The model under review builds one solid part; all positions refer to its coordinate system, in mm. Face numbers are marked on the shaded views. A direction names the side the tool comes from. Round coordinates to 2 decimals unless told otherwise and drop trailing zeros. Loops run counter-clockwise (first coordinate to the right, second up) from the corner with the lowest first, then second, coordinate; pieces in that order, holes last. Notation, with made-up numbers: M 48.25,52.25 L 60.25,52.25 A15 cw 60.25,81.25 Z; hole C 85.5,13.25 d8. An arc over 180 degrees is marked long. Answer as a JSON object with one key per item and string values. Group by question number.
Item 1: To check wall thickness, follow line 1 (Y direction, x = 15.5, z = 11); line 2 (X direction, y = -7.5, z = -13.5); line 3 (Z direction, x = 50, y = -35). State the ranges of each line that lie inside material, in increasing order.
Item 2: Insertion check: P1, Ø20, axis at y = -24.43, z = 34.69, coming from the +X side; P2, Ø23, axis at x = 7.5, y = -34, coming from the +Z side; P3, Ø2, axis at x = 16, y = -1.5, coming from the +Z side. Each pin has a flat end and moves straight along its axis. Give the tip position at first contact, or say it passes through.
Item 3: Consider section A-A (z = -2.5). Give the boundary of the cut face in (x, y).
Item 4: The part is to be moulded in two halves that separate along X. For the marked faces 3, 4 and 5, say which applies: +X half, -X half, draft (parallel to the pull), parting line (faces both ways), or undercut.
Item 5: Consider section D-D (z = 33). Give the boundary of the cut face in (x, y).
Item 6: Tool access review of the marked faces 1 and 2: name each direction out of +Z, -Z, +X, -X, +Y, -Y from which nothing blocks a thin tool from reaching the whole face with its end or side.
Item 7: Consider section C-C (x = 9.5). Give the boundary of the cut face in (y, z), and give its area (3 significant figures).
Item 8: Consider section B-B (y = -28.5). Give the boundary of the cut face in (x, z).
```python
from build123d import *

# Parameters (mm, degrees)
F1_DEPTH = 50.8
F2_T     = -2.54
F3_R     = 6.296308
F4_DEPTH = 322.58


with BuildPart() as f1:
    # F0 (on Front) → F1 (new body)
    with BuildSketch(Plane.XZ):
        Polygon((-25.901856, 44.70605), (-47.471371, 44.70605), (-47.471371, -22.952178), (64.985082, -22.952178), (64.985082, 44.70605), (46.365242, 44.70605), (46.365242, 21.47734), (-25.901856, 21.47734), align=None)
    extrude(amount=F1_DEPTH)

    # F2
    f2_openings = [f1.faces().sort_by_distance(p)[0] for p in [
        (10.231693, -25.4, 21.47734),
        (-36.686613, -25.4, 44.70605),
        (55.675162, -25.4, 44.70605),
        (46.365242, -25.4, 33.091695),
        (-25.901856, -25.4, 33.091695),
    ]]
    offset(amount=F2_T, openings=f2_openings)

    # F3 (on face) → F4 (cut)
    with BuildSketch(Plane(origin=(-47.471371, 0, 0), x_dir=(0, -1, 0), z_dir=(-1, 0, 0))):
        with Locations((24.432799, 34.693193)):
            Circle(F3_R)
    extrude(amount=-F4_DEPTH, mode=Mode.SUBTRACT)


solid = f1.part
```
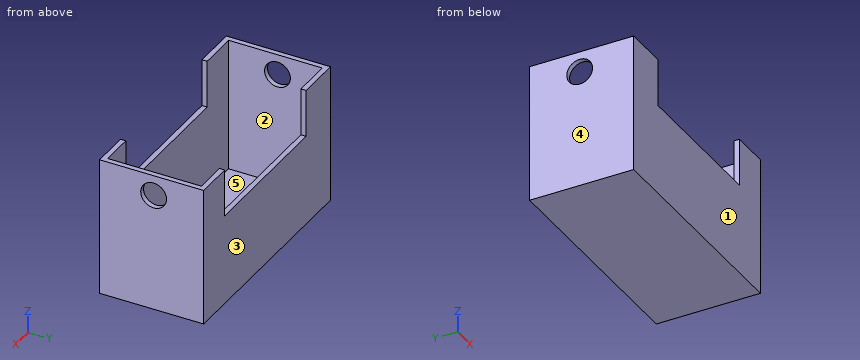
Geometry results:
{
 "1": {"line 1": "y = -50.8 to -48.26, -2.54 to 0", "line 2": "x = -47.47 to -44.93, 62.45 to 64.99", "line 3": "z = -22.95 to -20.41"},
 "2": {"P1": "stops at x = 64.99", "P2": "stops at z = -20.41", "P3": "stops at z = 21.48"},
 "3": {"outline": "M -47.47,-50.8 L 64.99,-50.8 L 64.99,0 L -47.47,0 Z; hole M -44.93,-48.26 L 62.45,-48.26 L 62.45,-2.54 L -44.93,-2.54 Z"},
 "4": {"face 3": "draft", "face 4": "-X half", "face 5": "undercut"},
 "5": {"outline": "M -47.47,-50.8 L -25.9,-50.8 L -25.9,-48.26 L -44.93,-48.26 L -44.93,-30.5 L -47.47,-30.5 Z; M -47.47,-18.37 L -44.93,-18.37 L -44.93,-2.54 L -25.9,-2.54 L -25.9,0 L -47.47,0 Z; M 46.37,-50.8 L 64.99,-50.8 L 64.99,-30.5 L 62.45,-30.5 L 62.45,-48.26 L 46.37,-48.26 Z; M 46.37,-2.54 L 62.45,-2.54 L 62.45,-18.37 L 64.99,-18.37 L 64.99,0 L 46.37,0 Z"},
 "6": {"face 1": "+Z, -Z, +X, -X, -Y", "face 2": "+Z"},
 "7": {"outline": "M -50.8,-22.95 L 0,-22.95 L 0,21.48 L -2.54,21.48 L -2.54,-20.41 L -48.26,-20.41 L -48.26,21.48 L -50.8,21.48 Z", "area": "342 mm^2"},
 "8": {"outline": "M -47.47,-22.95 L 64.99,-22.95 L 64.99,29.89 L 62.45,29.89 L 62.45,-20.41 L -44.93,-20.41 L -44.93,29.89 L -47.47,29.89 Z; M -47.47,39.5 L -44.93,39.5 L -44.93,44.71 L -47.47,44.71 Z; M 62.45,39.5 L 64.99,39.5 L 64.99,44.71 L 62.45,44.71 Z"}
}
